from build123d import *

# Parameters (mm, degrees)
F1_DEPTH     = 6.35
F2_R         = 3.175
F3_R         = 3.175
F4_DEPTH     = 2.54
F6_DEPTH     = 2.032
F7_T1_DEPTH  = 7.9826274972
F8_R         = 3.175
F9_R         = 2.0828
F10_DEPTH    = 4.7625
F12_DEPTH    = 1.016
F13_R        = 3.17499
F14_R        = 1.5875
F15_DEPTH    = 1.016
F19_DEPTH    = 6.351
F20_T1_DEPTH = 9.3839178422
F20_T3_DEPTH = 10.5760872304
F20_T5_DEPTH = 8.4107682306
F25_DEPTH    = 63.5


# Not quite as in the source:
# - a fillet or chamfer that OpenCascade refuses, or shapes differently, is made with other operations: its cross-section is extruded or revolved along the edge and cut away or added
# - a fillet or chamfer is up to 0.001 mm smaller than in the source, because OpenCascade refuses the exact size
# - a feature of the source that left no trace in its solid (it failed there, or was rolled back) is left out


with BuildPart() as f1:
    # F0 (on Top) → F1 (new body)
    with BuildSketch(Plane.XY):
        with BuildLine():
            ThreePointArc((25.4, -20.6375), (30.1625, 0), (25.4, 20.6375))
            Line((25.4, 20.6375), (-25.4, 20.6375))
            ThreePointArc((-25.4, 20.6375), (-30.1625, 0), (-25.4, -20.6375))
            Line((-25.4, -20.6375), (25.4, -20.6375))
        make_face()
    extrude(amount=F1_DEPTH)

    # F2
    f2_edges = [f1.edges().sort_by_distance(p)[0] for p in [
        (-25.4, 20.6375, 3.175),
        (-25.4, -20.6375, 3.175),
        (25.4, -20.6375, 3.175),
        (25.4, 20.6375, 3.175),
    ]]
    fillet(f2_edges, radius=F2_R)

    # F3 (on face) → F4 (join)
    with BuildSketch(Plane.XY.offset(6.35)):
        with Locations((-19.1135, 0)):
            Circle(F3_R)
    extrude(amount=F4_DEPTH)

    # F5 (on face) → F6 (join)
    with BuildSketch(Plane.XY.offset(6.35)):
        with BuildLine():
            ThreePointArc((25.7962114887, 10.16), (24.151933107, 15.5254784859), (21.8369283945, 20.6375))
            Line((21.8369283945, 20.6375), (-16.002, 20.6375))
            ThreePointArc((-16.002, 20.6375), (-13.4865218815, 13.6398781095), (-12.0195455914, 6.35))
            Line((-12.0195455914, 6.35), (-11.2165052403, 9.2309969527))
            ThreePointArc((-11.2165052403, 9.2309969527), (-10.7612010879, 9.9014262529), (-9.9931405857, 10.16))
            Line((-9.9931405857, 10.16), (25.7962114887, 10.16))
        make_face()
    extrude(amount=F6_DEPTH)

    # F7: fillet of radius 0.508 on 1 edges, made by hand

    # F7_s2 → F7_t1 (cut)
    with BuildSketch(Plane.XY.offset(6.35)):
        with BuildLine():
            ThreePointArc((-12.3702984959, 8.6923219718), (-11.8951499479, 8.2718785653), (-11.3804445383, 8.6428464104))
            Line((-11.3804445383, 8.6428464104), (-12.0195455914, 6.35))
            ThreePointArc((-12.0195455914, 6.35), (-12.1812694874, 7.523205399), (-12.3702984959, 8.6923219718))
        make_face()
    extrude(amount=F7_T1_DEPTH, mode=Mode.SUBTRACT)

    # F8
    f8_edges = [f1.edges().sort_by_distance(p)[0] for p in [
        (21.836928, 20.6375, 7.366),
    ]]
    fillet(f8_edges, radius=F8_R)

    # F9 (on face) → F10 (cut)
    with BuildSketch(Plane.XY.offset(8.89)):
        with Locations((-19.1135, 0)):
            Circle(F9_R)
    extrude(amount=-F10_DEPTH, mode=Mode.SUBTRACT)

    # F11 (on face) → F12 (cut)
    with BuildSketch(Plane.XY.offset(6.35)):
        with BuildLine():
            ThreePointArc((-11.7204239002, 3.175), (-11.6211080672, 0), (-11.7204239002, -3.175))
            Line((-11.7204239002, -3.175), (20.0295760998, -3.175))
            Line((20.0295760998, -3.175), (20.0295760998, 3.175))
            Line((20.0295760998, 3.175), (-11.7204239002, 3.175))
        make_face()
    extrude(amount=-F12_DEPTH, mode=Mode.SUBTRACT)

    # F13 (radius 3.175 in the source; OpenCascade refuses exactly that, so slightly less here)
    f13_edges = [f1.edges().sort_by_distance(p)[0] for p in [
        (20.029576, 3.175, 5.842),
        (20.029576, -3.175, 5.842),
    ]]
    fillet(f13_edges, radius=F13_R)

    # F14 (on face) → F15 (join, through all)
    with BuildSketch(Plane.XY.offset(5.334)):
        with Locations((16.8545760998, 0)):
            Circle(F14_R)
    extrude(amount=F15_DEPTH)

    # F18 (on face) → F19 (cut, through all)
    with BuildSketch(Plane.XY.offset(6.35)):
        with BuildLine():
            Line((8.1267993519, -20.6375), (23.3667993519, -20.6375))
            ThreePointArc((23.3667993519, -20.6375), (15.7467993519, -18.0975), (8.1267993519, -20.6375))
        make_face()
        with BuildLine():
            Line((-7.1132006481, -20.6375), (8.1267993519, -20.6375))
            ThreePointArc((8.1267993519, -20.6375), (0.5067993519, -18.0975), (-7.1132006481, -20.6375))
        make_face()
        with BuildLine():
            Line((-22.3532006481, -20.6375), (-7.1132006481, -20.6375))
            ThreePointArc((-7.1132006481, -20.6375), (-14.7332006481, -18.0975), (-22.3532006481, -20.6375))
        make_face()
    extrude(amount=-F19_DEPTH, mode=Mode.SUBTRACT)

    # F20: fillet of radius 1.27 on 4 edges, made by hand

    # F20_s2 → F20_t1 (cut)
    with BuildSketch(Plane.XY.offset(-1.5169589211)):
        with BuildLine():
            ThreePointArc((23.9708158767, -20.5796179073), (23.4664541239, -20.5753299276), (23.0035373612, -20.3750620187))
            Line((23.0035373612, -20.3750620187), (22.9890237709, -20.3959070588))
            ThreePointArc((22.9890237709, -20.3959070588), (23.1714765643, -20.5252240374), (23.3515593519, -20.65782))
            Line((23.3515593519, -20.65782), (23.3667993519, -20.6629))
            ThreePointArc((23.3667993519, -20.6629), (23.6726182662, -20.648255005), (23.9756478567, -20.6045540651))
            Line((23.9756478567, -20.6045540651), (23.9708158767, -20.5796179073))
        make_face()
    extrude(amount=F20_T1_DEPTH, mode=Mode.SUBTRACT)

    # F20_s4 → F20_t3 (cut)
    with BuildSketch(Plane.XY.offset(-2.1130436152)):
        with BuildLine():
            ThreePointArc((8.8195315833, -20.1532329387), (8.1267993519, -20.3587978512), (7.4340671204, -20.1532329387))
            Line((7.4340671204, -20.1532329387), (7.4202124758, -20.1745216404))
            ThreePointArc((7.4202124758, -20.1745216404), (7.7699369678, -20.410377341), (8.1115593519, -20.65782))
            Line((8.1115593519, -20.65782), (8.1420393519, -20.65782))
            ThreePointArc((8.1420393519, -20.65782), (8.4836617359, -20.410377341), (8.8333862279, -20.1745216404))
            Line((8.8333862279, -20.1745216404), (8.8195315833, -20.1532329387))
        make_face()
        with BuildLine():
            ThreePointArc((-6.4204684167, -20.1532329387), (-7.1132006481, -20.3587978512), (-7.8059328796, -20.1532329387))
            Line((-7.8059328796, -20.1532329387), (-7.8197875242, -20.1745216404))
            ThreePointArc((-7.8197875242, -20.1745216404), (-7.4700630322, -20.410377341), (-7.1284406481, -20.65782))
            Line((-7.1284406481, -20.65782), (-7.0979606481, -20.65782))
            ThreePointArc((-7.0979606481, -20.65782), (-6.7563382641, -20.410377341), (-6.4066137721, -20.1745216404))
            Line((-6.4066137721, -20.1745216404), (-6.4204684167, -20.1532329387))
        make_face()
    extrude(amount=F20_T3_DEPTH, mode=Mode.SUBTRACT)

    # F20_s6 → F20_t5 (cut)
    with BuildSketch(Plane.XY.offset(-1.0303841153)):
        with BuildLine():
            ThreePointArc((-22.0351532703, -20.4066892562), (-22.382433504, -20.5784970549), (-22.7653542821, -20.6376))
            Line((-22.7653542821, -20.6376), (-22.7653542821, -20.663))
            ThreePointArc((-22.7653542821, -20.663), (-22.5592774651, -20.6629), (-22.3532006481, -20.6629))
            Line((-22.3532006481, -20.6629), (-22.3379606481, -20.65782))
            ThreePointArc((-22.3379606481, -20.65782), (-22.1801756491, -20.5413775117), (-22.0205492501, -20.4274710413))
            Line((-22.0205492501, -20.4274710413), (-22.0351532703, -20.4066892562))
        make_face()
    extrude(amount=F20_T5_DEPTH, mode=Mode.SUBTRACT)

    # F21 (on Front) → F23 (revolve, cut)
    with BuildSketch(Plane.XZ):
        Polygon((26.9875, 4.7625), (26.9875, 3.175), (30.1625, 3.175), (30.1625, 6.35), (28.575, 6.35), (28.575, 4.7625), align=None)
    revolve(axis=Axis((-20.6375, 0, 8.7874885648), (0, 0, 1)), mode=Mode.SUBTRACT)

    # F24 (on Right) → F25 (cut, symmetric)
    with BuildSketch(Plane.YZ):
        Polygon((15.875, 3.175), (20.6375, 3.175), (20.6375, 8.382), (17.4625, 8.382), (17.4625, 4.7625), (15.875, 4.7625), align=None)
        Polygon((-15.875, 4.7625), (-17.4625, 4.7625), (-17.4625, 8.382), (-20.6375, 8.382), (-20.6375, 3.175), (-15.875, 3.175), align=None)
    extrude(amount=F25_DEPTH, both=True, mode=Mode.SUBTRACT)


solid = f1.part
Input: part model. Units: mm. Frame: model coordinates. A direction names the side the tool comes from. Give positions to 0.01 mm unless a question says otherwise; leave off trailing zeros.
Q1. Pull-direction query (X, two-part tool) for faces 6 (the face through (9, -17, 4.762)), 7 (the face through (-13.364, 13.191, 7.352)), 8 (the face through (-14.9, -18.1, 1.6)), 9 (the face through (8.14, -20.36, 1.57)); classes: pulls with the +X half, pulls with the -X half, needs draft (parallel to the pull), parting line crosses it, or undercut.
Q2. First-contact query: P1, Ø8, axis at x = -16, y = 10, coming from the -Z side; P2, Ø5, axis at x = 0, z = 7.5, coming from the +Y side; P3, Ø1, axis at x = -1, z = 2.5, coming from the -Y side; P4, Ø4, axis at y = 4.5, z = 7, coming from the -X side. Flat tips, straight axial feed; report the tip coordinate or a pass-through.
Q3. Set-up query: faces 1 (the face through (6, 17, 3.175)), 2 (the face through (4, 0, 5.334)), 3 (the face through (-2, 15.875, 4)), 4 (the face through (0, -17.462, 6)), 5 (the face through (28.574, -0.25, 5.545)). Return all of +Z, -Z, +X, -X, +Y, -Y with unobstructed straight access to the full face (end or side cutting, diameter ignored); none if empty.
Q4. Material intervals for probe 1 along Y at (x, z) = (7, 5.75) (1 decimal); probe 2 along Z at (x, y) = (18.5, 14); probe 3 along Y at (x, z) = (13.5, 8.25), sorted ascending.
Filled in:
1. face 6: needs draft
1. face 7: pulls with the -X half
1. face 8: undercut
1. face 9: undercut
2. P1: stops at z = 0
2. P2: stops at y = 17.46
2. P3: stops at y = -18.26
2. P4: stops at x = -30.09
3. face 1: +X
3. face 2: +Z
3. face 3: +X, -X, +Y
3. face 4: +Z, +X, -X, -Y
3. face 5: +Z, +X
4. probe 1: y = -17.5 to -3.2, 3.2 to 17.5
4. probe 2: z = 0 to 8.38
4. probe 3: y = 10.16 to 17.46
